For this review, take the finished solid that the model builds, in its own axes (mm). Face numbers are marked on the shaded views. A direction names the side the tool comes from. Round coordinates to 2 decimals unless told otherwise and drop trailing zeros. Loops run counter-clockwise (first coordinate to the right, second up) from the corner with the lowest first, then second, coordinate; pieces in that order, holes last.
1. Consider section D-D on z = 69.5. State the section outline as (x, y) points.
2. Clearance check with flat-ended pins moving along their axes: pin 1 Ø2.5 at (y, z) = (7.5, 65) entering from -X; pin 2 Ø4 at (x, z) = (0, 10) entering from -Y. State where each tip first meets the part, or that it passes through.
3. To check wall thickness, follow line 1 along X through (y, z) = (9, 8); line 2 along X through (y, z) = (-14.8, 30); line 3 along Y through (x, z) = (4.75, 5.5). State the ranges of each line that lie inside material, in increasing order.
4. Consider section A-A on y = -4. State the section outline as (x, z) points, then the cut area to 3 significant figures.
5. Draft analysis for pull direction X (two halves, no side actions). For the marked faces 1, 2, 3 and 4, state which applies: released by +X, released by -X, zero draft, split by the parting line, or undercut.
6. Tool access review of the marked faces 5 and 6: name each direction out of +Z, -Z, +X, -X, +Y, -Y from which nothing blocks a thin tool from reaching the whole face with its end or side.
7. Consider section B-B on z = 55. State the section outline as (x, y) points.
8. Consider section C-C on x = 0. State how many separate pieces and enclosed holes the cut face has, then the cut area to 3 significant figures.
Autodesk Inventor part; units mm, degrees
ref_plane "YZ Plane" through (0, 0, 0) normal (1, 0, 0) x (0, 1, 0)
ref_plane "XZ Plane" through (0, 0, 0) normal (0, 1, 0) x (-1, 0, 0)
ref_plane "XY Plane" through (0, 0, 0) normal (0, 0, 1) x (1, 0, 0)
sketch "スケッチ1" plane through (0, 0, 0) normal (0, 0, 1) x (1, 0, 0)
  line L0 (7.5, 15) -> (-7.5, 15)
  line L1 (-7.5, 15) -> (-7.5, -15)
  line L2 (-7.5, -15) -> (7.5, -15)
  line L3 (7.5, -15) -> (7.5, 15)
  line L4 (7.5, 15) -> (-7.5, -15) construction
  line L5 (-7.5, 15) -> (7.5, -15) construction
  line L6 (-6.5, 14) -> (6.5, 14)
  line L7 (6.5, 14) -> (6.5, -14)
  line L8 (6.5, -14) -> (-6.5, -14)
  line L9 (-6.5, -14) -> (-6.5, 14)
  point P0 (0, 0)
  dimension "d0" = 15
  dimension "d1" = 30
  dimension "d2" = 1
extrude "押し出し1" add sketch "スケッチ1" along normal blind 115
sketch "スケッチ2" plane through (-7.5, 15, 0) normal (0, 1, 0) x (1, 0, 0)
  circle A0 centre (7.5, -10) radius 1.6
  circle A1 centre (7.5, -20) radius 1.6
  circle A2 centre (7.5, -30) radius 1.6
  circle A3 centre (7.5, -105) radius 1.6
  circle A4 centre (7.5, -95) radius 1.6
  circle A5 centre (7.5, -85) radius 1.6
  line L0 (15, -115) -> (0, -115)
  line L1 (15, 0) -> (0, 0)
  point P0 (7.5, 0)
  point P1 (7.5, 0)
  dimension "d5" = 3.2
  dimension "d6" = 3.2
  dimension "d7" = 3.2
  dimension "d8" = 3.2
  dimension "d9" = 3.2
  dimension "d10" = 3.2
  dimension "d11" = 10
  dimension "d12" = 10
  dimension "d13" = 10
  dimension "d14" = 10
  dimension "d15" = 10
  dimension "d16" = 10
extrude "押し出し2" cut sketch "スケッチ2" against normal through all
sketch "スケッチ3" plane through (7.5, -15, 0) normal (1, 0, 0) x (0, 0, -1)
  circle A0 centre (-65, 22.5) radius 1.6
  circle A1 centre (-55, 22.5) radius 1.6
  circle A2 centre (-45, 22.5) radius 1.6
  line L0 (0, 0) -> (0, 30)
  line L1 (0, 30) -> (-115, 30)
  point P0 (0, 15)
  dimension "d19" = 3.2
  dimension "d20" = 3.2
  dimension "d21" = 3.2
  dimension "d22" = 10
  dimension "d23" = 10
  dimension "d24" = 45
  dimension "d25" = 7.5
extrude "押し出し3" cut sketch "スケッチ3" against normal through all
properties part number "オムニ_角柱7" material "アルミニウム 6061"
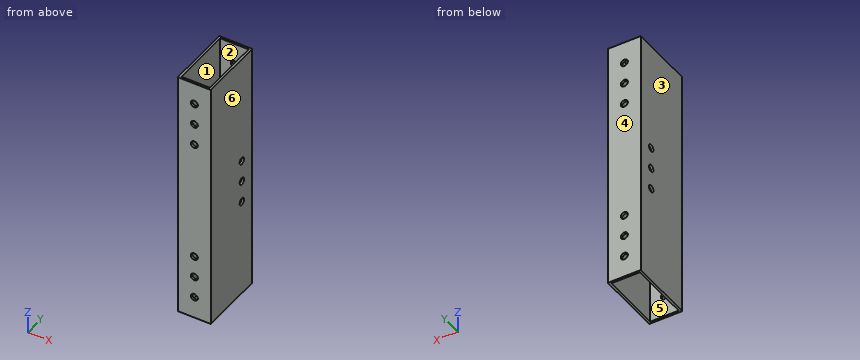
Resolved:
1. outline: (-7.5, -15) - (7.5, -15) - (7.5, 15) - (-7.5, 15) - close; hole (-6.5, -14) - (6.5, -14) - (6.5, 14) - (-6.5, 14) - close
2. pin 1: passes through
2. pin 2: stops at y = -15
3. line 1: x = -7.5 to -6.5, 6.5 to 7.5
3. line 2: x = -7.5 to -1.6, 1.6 to 7.5
3. line 3: y = -15 to -14, 14 to 15
4. outline: (-7.5, 0) - (-6.5, 0) - (-6.5, 115) - (-7.5, 115) - close; (6.5, 0) - (7.5, 0) - (7.5, 115) - (6.5, 115) - close
4. area: 230 mm2
5. face 1: undercut
5. face 2: undercut
5. face 3: released by -X
5. face 4: zero draft
6. face 5: +Z, -Z
6. face 6: +Z, -Z, +X, +Y, -Y
7. outline: (-7.5, -15) - (7.5, -15) - (7.5, 5.9) - (6.5, 5.9) - (6.5, -14) - (-6.5, -14) - (-6.5, 5.9) - (-7.5, 5.9) - close; (-7.5, 9.1) - (-6.5, 9.1) - (-6.5, 14) - (6.5, 14) - (6.5, 9.1) - (7.5, 9.1) - (7.5, 15) - (-7.5, 15) - close
8. separate pieces: 14
8. enclosed holes: 0
8. area: 192 mm2
